```python
from build123d import *

# Parameters (mm, degrees)
SKETCH1_W                       = 58
SKETCH1_H                       = 35
BOSS_EXTRUDE2_DEPTH             = 2
M3X0_5_TAPPED_HOLE3_D           = 2.5
M3X0_5_TAPPED_HOLE3_CSINK_D     = 3.05
M3X0_5_TAPPED_HOLE3_CSINK_ANGLE = 90
CUT_EXTRUDE1_DEPTH              = 3


with BuildPart() as part:
    # Sketch1 → Boss-Extrude2 (new body)
    with BuildSketch(Plane.XY):
        Rectangle(SKETCH1_W, SKETCH1_H)
    extrude(amount=BOSS_EXTRUDE2_DEPTH)

    # M3x0.5 Tapped Hole3 (through all)
    with Locations(Plane.XY.offset(2)):
        with Locations((-23, 12.5), (-3, 12.5), (16.8, 12.5), (16.8, -6.5), (-23, -1.5)):
            CounterSinkHole(M3X0_5_TAPPED_HOLE3_D / 2, M3X0_5_TAPPED_HOLE3_CSINK_D / 2, counter_sink_angle=M3X0_5_TAPPED_HOLE3_CSINK_ANGLE)

    # Sketch11 → Cut-Extrude1 (cut, through all)
    with BuildSketch(Plane.XY.offset(2)):
        with BuildLine():
            ThreePointArc((-8.204545455, -3.514584349), (-11.5, -6.5), (-8.204545455, -9.485415651))
            ThreePointArc((-8.204545455, -9.485415651), (3, -6.5), (-8.204545455, -3.514584349))
        make_face()
    extrude(amount=-CUT_EXTRUDE1_DEPTH, mode=Mode.SUBTRACT)


solid = part.part
```
Input: part model. Units: mm. Frame: model coordinates. Coordinates: 2 decimals unless noted, no trailing zeros. Loops run counter-clockwise (first coordinate to the right, second up) from the corner with the lowest first, then second, coordinate; pieces in that order, holes last. Notation, with made-up numbers: M 22.25,81 L 27.25,81 A19 ccw 27.25,88 Z; hole C 74.25,76.25 d6. An arc over 180 degrees is marked long. Use a Markdown table: item, result. Add a question column.
1) Section D-D, the plane x = -3. Return the cut outline in (y, z) (3 decimals).
2) Section B-B, the plane x = 16.8. Return the cut outline in (y, z) (3 decimals).
3) Line query: L1, parallel to Y at x = -23, z = 0.9; L2, parallel to X at y = -6.5, z = 0.6; L3, parallel to Y at x = -3, z = 0.6. Output: solid intervals per line, ascending. Write a range as from..to.
4) Section A-A, the plane y = 12.5. Return the cut outline in (x, z) (3 decimals).
5) Pin query (flat end, axial travel): P1, Ø4, axis at x = -23, y = -1.5, coming from the +Z side; P2, Ø2, axis at x = 16.8, y = -6.5, coming from the +Z side. Return the tip coordinate at first contact, or that it passes through.
6) Draft query along Y for faces 1 (the flat face through (0, -17.5, 1)), 2 (the flat face through (29, 0, 1)), 3 (the cylindrical face through (2.996, -6.72, 1.014)). Return one class per face: +Y half, -Y half, draft (parallel to the pull), parting line (faces both ways), or undercut.
7) Section C-C, the plane y = -6.5. Return the cut outline in (x, z) (3 decimals), plus the area to 3 significant figures.
Answer below:
| question | item | result |
|---|---|---|
| 1 | outline | M -17.5,0 L -12.5,0 L -12.5,2 L -17.5,2 Z; M -0.5,0 L 11.25,0 L 11.25,1.725 L 10.975,2 L -0.5,2 Z; M 13.75,0 L 17.5,0 L 17.5,2 L 14.025,2 L 13.75,1.725 Z |
| 2 | outline | M -17.5,0 L -7.75,0 L -7.75,1.725 L -8.025,2 L -17.5,2 Z; M -5.25,0 L 11.25,0 L 11.25,1.725 L 10.975,2 L -4.975,2 L -5.25,1.725 Z; M 13.75,0 L 17.5,0 L 17.5,2 L 14.025,2 L 13.75,1.725 Z |
| 3 | L1 | -17.5..-2.75, -0.25..11.25, 13.75..17.5 |
| 3 | L2 | -29..-11.5, 3..15.55, 18.05..29 |
| 3 | L3 | -17.5..-12.5, -0.5..11.25, 13.75..17.5 |
| 4 | outline | M -29,0 L -24.25,0 L -24.25,1.725 L -24.525,2 L -29,2 Z; M -21.75,0 L -4.25,0 L -4.25,1.725 L -4.525,2 L -21.475,2 L -21.75,1.725 Z; M -1.75,0 L 15.55,0 L 15.55,1.725 L 15.275,2 L -1.475,2 L -1.75,1.725 Z; M 18.05,0 L 29,0 L 29,2 L 18.325,2 L 18.05,1.725 Z |
| 5 | P1 | z = 2 |
| 5 | P2 | through |
| 6 | face 1 | -Y half |
| 6 | face 2 | draft |
| 6 | face 3 | undercut |
| 7 | outline | M -29,0 L -11.5,0 L -11.5,2 L -29,2 Z; M 3,0 L 15.55,0 L 15.55,1.725 L 15.275,2 L 3,2 Z; M 18.05,0 L 29,0 L 29,2 L 18.325,2 L 18.05,1.725 Z |
| 7 | area | 81.9 mm2 |
